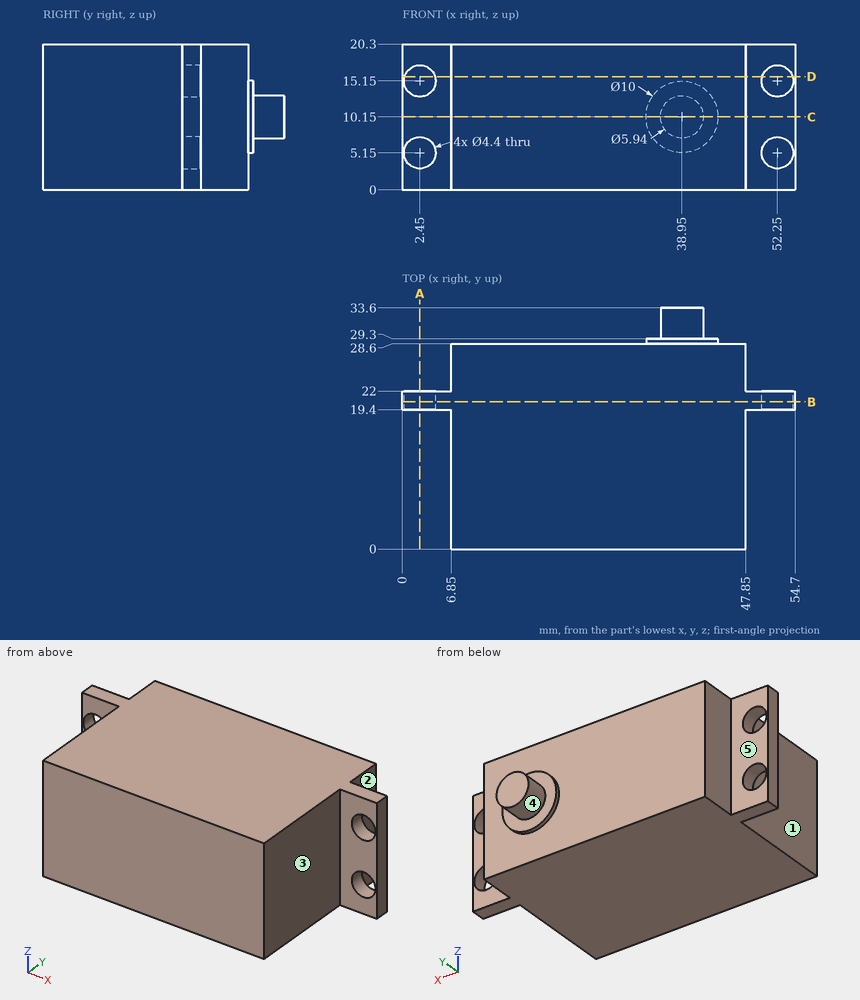
Input: dimensioned drawing with shaded views. Units: mm. Origin: part minimum x, y, z. A direction names the side the tool comes from. Round coordinates to 2 decimals unless told otherwise and drop trailing zeros. Order: outer loops, then holes, each group sorted by start corner. A loop starts at its lowest first (then second) coordinate and runs counter-clockwise, first axis right, second up. Notation, with made-up numbers: (11, 53) -> (63, 53) arc R15 cw to (63, 75) -> close; hole circle Ø1 at (45, 76). An arc over 180 degrees is marked (long way). Put each result on its own line as item: value. Start each with the question number.
Q1. Section D-D on z = 15.75. Return the cut outline in (x, y).
Q2. Reachability of the marked faces 1, 2, 3, 4 and 5 from +Z, -Z, +X, -X, +Y, -Y: full face, straight path, thin tool, end or side. Return the list, or none.
Q3. Section B-B on y = 20.5. Return the cut outline in (x, z), and give its area (3 significant figures).
Q4. First-contact query: pin 1 (7.5 mm diameter, centred on x = 2, z = 15, fed in from -Y); pin 2 (5.5 mm diameter, centred on y = 26, z = 12.5, fed in from -X); pin 3 (6 mm diameter, centred on y = 9, z = 13, fed in from +X); pin 4 (2.5 mm diameter, centred on x = 52.25, z = 15.15, fed in from +Y). Flat tips, straight axial feed; report the tip coordinate or a pass-through.
Q5. Section A-A on x = 2.45. Return the cut outline in (y, z), and give its area (3 significant figures).
Q6. Section C-C on z = 10.15. Return the cut outline in (x, y).
Q7. Line query: probe 1 along X at (y, z) = (21.4, 5.15); probe 2 along Z at (x, y) = (52, 20); probe 3 along X at (y, z) = (5.5, 6.75). Output: solid intervals per line, ascending.
Ans:
1. outline: (0, 19.4) -> (0.33, 19.4) -> (0.33, 22) -> (0, 22) -> close; (4.57, 19.4) -> (6.85, 19.4) -> (6.85, 0) -> (47.85, 0) -> (47.85, 19.4) -> (50.13, 19.4) -> (50.13, 22) -> (47.85, 22) -> (47.85, 28.6) -> (6.85, 28.6) -> (6.85, 22) -> (4.57, 22) -> close; (54.37, 19.4) -> (54.7, 19.4) -> (54.7, 22) -> (54.37, 22) -> close
2. face 1: +Z, -Z, -X, -Y
2. face 2: +Z, -Z, +X, +Y
2. face 3: +Z, -Z, +X, -Y
2. face 4: +Y
2. face 5: +Z, -Z, -X, +Y
3. outline: (0, 0) -> (54.7, 0) -> (54.7, 20.3) -> (0, 20.3) -> close; hole circle Ø4.4 at (2.45, 5.15); hole circle Ø4.4 at (2.45, 15.15); hole circle Ø4.4 at (52.25, 5.15); hole circle Ø4.4 at (52.25, 15.15)
3. area: 1,050 mm2
4. pin 1: stops at y = 19.4
4. pin 2: stops at x = 6.85
4. pin 3: stops at x = 47.85
4. pin 4: passes through
5. outline: (19.4, 0) -> (22, 0) -> (22, 2.95) -> (19.4, 2.95) -> close; (19.4, 7.35) -> (22, 7.35) -> (22, 12.95) -> (19.4, 12.95) -> close; (19.4, 17.35) -> (22, 17.35) -> (22, 20.3) -> (19.4, 20.3) -> close
5. area: 29.9 mm2
6. outline: (0, 19.4) -> (6.85, 19.4) -> (6.85, 0) -> (47.85, 0) -> (47.85, 19.4) -> (54.7, 19.4) -> (54.7, 22) -> (47.85, 22) -> (47.85, 28.6) -> (43.95, 28.6) -> (43.95, 29.3) -> (41.92, 29.3) -> (41.92, 33.6) -> (35.98, 33.6) -> (35.98, 29.3) -> (33.95, 29.3) -> (33.95, 28.6) -> (6.85, 28.6) -> (6.85, 22) -> (0, 22) -> close
7. probe 1: x = 0 to 0.25, 4.65 to 50.05, 54.45 to 54.7
7. probe 2: z = 0 to 2.96, 7.34 to 12.96, 17.34 to 20.3
7. probe 3: x = 6.85 to 47.85
